Read the model definition and answer for the solid it produces. Units are mm, in the model's axes. A direction names the side the tool comes from. Give positions to 0.01 mm unless a question says otherwise; leave off trailing zeros. Write each loop counter-clockwise with the first axis right and the second up, starting at its lowest first coordinate (ties: lowest second). Pieces come first, ordered by that corner, then holes. Notation, with made-up numbers: (32, 88) -> (78, 88) arc R15 cw to (78, 115) -> close; hole circle Ø7 at (31, 74). An arc over 180 degrees is marked (long way). Use a Markdown table: item, result.
from build123d import *

# Parameters (mm, degrees)
F0_R            = 50.8
F1_DEPTH        = 25.4
F3_DEPTH        = 25.4
F3_COPIES_COUNT = 36


# Not quite as in the source:
# - a pattern or mirror of a feature is missing from the dataset's text; its kind, count and spacing are read off the source's solid


with BuildPart() as f1:
    # F0 (on Front) → F1 (new body)
    with BuildSketch(Plane.XZ):
        Circle(F0_R)
    extrude(amount=F1_DEPTH)

    # F2 (on Front) → F3 (join, through all)
    with BuildSketch(Plane.XZ):
        Polygon((4.4275117316, 50.6066906631), (0, 55.88), (-4.4275117316, 50.6066906631), align=None)
    f3 = extrude(amount=F3_DEPTH)

    # F3_copies: F3 ×36 about axis
    f3_copies_axis = Axis((0, 0, 0), (0, 1, 0))
    for i in range(1, F3_COPIES_COUNT):
        add(f3.rotate(f3_copies_axis, i * 360 / F3_COPIES_COUNT))


solid = f1.part
Item 1: A tool of negligible diameter and unlimited length cuts with its end or side. For faces 1 (the face through (16.088, -12.522, -50.765)), 2 (the face through (42.22, -12.52, -32.58)), 3 (the face through (20.307, -12.522, 49.23)), 4 (the face through (-52.79, -12.52, -7.03)), from which of +Z, -Z, +X, -X, +Y, -Y can it reach the whole face along a straight path? Write none if from no direction.
Return value:
| item | result |
|---|---|
| face 1 | -Z, +Y, -Y |
| face 2 | +X, +Y, -Y |
| face 3 | +Z, +Y, -Y |
| face 4 | -X, +Y, -Y |
Item 2: A cutting plane is placed at B-B (x = -32). Give the vertices of the cut face in (y, z).
Return value:
| item | result |
|---|---|
| outline | (-25.4, -42.12) -> (0, -42.12) -> (0, 42.12) -> (-25.4, 42.12) -> close |
Item 3: Straight lines are drawn through the part: line 1 along X through (y, z) = (-15, 50); line 2 along Z through (x, y) = (49.5, -23.75); line 3 along Z through (x, y) = (-5.5, -1.5). For each, find the intervals that lie inside material, in ascending order. Write a range as [from, to].
Return value:
| item | result |
|---|---|
| line 1 | [-20.03, -14.76], [-12.61, 12.61], [14.76, 20.03] |
| line 2 | [-20.21, -13.89], [-12.9, 12.9], [13.89, 20.21] |
| line 3 | [-51.51, 51.51] |
Item 4: A cutting plane is placed at A-A (z = 38.5). Give the vertices of the cut face in (x, y).
Return value:
| item | result |
|---|---|
| outline | (-35.92, -25.4) -> (35.92, -25.4) -> (35.92, 0) -> (-35.92, 0) -> close |
Item 5: Each of these flat-tipped pins is pushed along its axis until it touches: P1, Ø3, axis at y = -17, z = -11, coming from the +X side; P2, Ø1.5, axis at x = -8, y = -10.5, coming from the -Z side; P3, Ø7.5, axis at y = -17, z = -38, coming from the -X side. Where does it stop, or does it pass through?
Return value:
| item | result |
|---|---|
| P1 | x = 55.03 |
| P2 | z = -54.23 |
| P3 | x = -42.81 |
Item 6: For a pull along X with two mould halves and no side action, classify faces 5 (the face through (-50.814, -12.522, 16.172)), 6 (the face through (-16.172, -12.522, -50.814)), 7 (the face through (45.05, -12.52, 28.53)) as +X half, -X half, draft (parallel to the pull), parting line (faces both ways), or undercut.
Return value:
| item | result |
|---|---|
| face 5 | -X half |
| face 6 | undercut |
| face 7 | +X half |
